Read the model definition and answer for the solid it produces. Units are mm, in the model's axes. A direction names the side the tool comes from. Coordinates: 2 decimals unless noted, no trailing zeros. Write each loop counter-clockwise with the first axis right and the second up, starting at its lowest first coordinate (ties: lowest second). Pieces come first, ordered by that corner, then holes. Notation, with made-up numbers: (64, 42) -> (102, 42) arc R23 cw to (102, 74) -> close; hole circle Ø3 at (-35, 27). An arc over 180 degrees is marked (long way). Return JSON: item names as keys, results as strings.
from build123d import *

# Parameters (mm, degrees)
F0_W           = 46.347648
F0_H           = 32.971419
F1_DEPTH       = 25
F3_D           = 5
F3_CSINK_D     = 10
F3_CSINK_ANGLE = 90
F5_D           = 5
F5_CBORE_D     = 10
F5_CBORE_DEPTH = 5


with BuildPart() as f1:
    # F0 (on Front) → F1 (new body)
    with BuildSketch(Plane.XZ):
        with Locations((47.167972, 16.485709)):
            Rectangle(F0_W, F0_H)
    extrude(amount=F1_DEPTH)

    # F3 (through all)
    with Locations(Plane.XZ.offset(25)):
        with Locations((44.375189, 15.056089)):
            CounterSinkHole(F3_D / 2, F3_CSINK_D / 2, counter_sink_angle=F3_CSINK_ANGLE)

    # F5 (through all)
    with Locations(Plane.YZ.offset(70.341796)):
        with Locations((-9.982947, 16.622152)):
            CounterBoreHole(F5_D / 2, F5_CBORE_D / 2, F5_CBORE_DEPTH)


solid = f1.part
1. A tool of negligible diameter and unlimited length cuts with its end or side. For faces 5 (the face through (47, -25, 20)), 6 (the face through (67.88, -10.63, 21.58)), from which of +Z, -Z, +X, -X, +Y, -Y can it reach the whole face along a straight path? Write none if from no direction.
Taken from the geometry:
{"face 5": "+Z, -Z, +X, -X, -Y", "face 6": "+X"}
2. For a pull along X with two mould halves and no side action, classify faces 1 (the face through (43.17, -22.62, 12.73)), 2 (the face through (43.22, -11.09, 12.84)), 3 (the face through (47, -12, 0)), 4 (the face through (65.342, -8, 14)) as +X half, -X half, draft (parallel to the pull), parting line (faces both ways), or undercut.
Taken from the geometry:
{"face 1": "undercut", "face 2": "undercut", "face 3": "draft", "face 4": "+X half"}
3. The part is cut by section A-A (y = -10.75). Determine the outline of the cut face in (x, z).
Taken from the geometry:
{"outline": "(23.99, 0) -> (70.34, 0) -> (70.34, 11.68) -> (65.34, 11.68) -> (65.34, 14.24) -> (46.74, 14.24) arc R2.5 cw to (42.01, 14.24) -> (23.99, 14.24) -> close; (23.99, 19) -> (65.34, 19) -> (65.34, 21.56) -> (70.34, 21.56) -> (70.34, 32.97) -> (23.99, 32.97) -> close"}
4. Consider L1, parallel to Y at x = 64.5, z = 16.5; L2, parallel to Y at x = 47.5, z = 17.5; L3, parallel to Z at x = 34.5, y = -11.75. Determine where each line is inside the solid, lowest interval first.
Taken from the geometry:
{"L1": "y = -25 to -12.48, -7.49 to 0", "L2": "y = -23.97 to -12.32, -7.64 to 0", "L3": "z = 0 to 14.85, 18.39 to 32.97"}
5. The part is cut by section B-B (x = 62.5). Determine the outline of the cut face in (y, z), then the cut area to 3 significant figures.
Taken from the geometry:
{"outline": "(-25, 0) -> (0, 0) -> (0, 32.97) -> (-25, 32.97) -> close; hole circle Ø5 at (-9.98, 16.62)", "area": "805 mm2"}
6. Flat-ended cylindrical pins translate along their axes: pin 1 Ø6 at (y, z) = (-9.98, 16.62) entering from +X; pin 2 Ø4.5 at (x, z) = (44.38, 15.06) entering from -Y. Find the tip coordinate at first contact, or state that the pin passes through.
Taken from the geometry:
{"pin 1": "stops at x = 65.34", "pin 2": "passes through"}
